Can you work these out from the drawing? Everything is in mm from the part's minimum corner. Round coordinates to 2 decimals unless told otherwise and drop trailing zeros. Write each loop counter-clockwise with the first axis right and the second up, starting at its lowest first coordinate (ties: lowest second). Pieces come first, ordered by that corner, then holes. Notation, with made-up numbers: (-39, 20.5) -> (14, 20.5) arc R28 ccw to (14, 49.5) -> close; hole circle Ø11 at (-11.5, 42.5). An arc over 180 degrees is marked (long way). One line per question, with ' | ' between items. Start each with the question number.
1. Imagine slicing it at B-B, the plane z = 50.8. List the corners of the cut face in (x, y) for me.
2. Imagine slicing it at D-D, the plane x = 64. List the corners of the cut face in (y, z) for me.
3. Imagine slicing it at A-A, the plane x = 38.1. List the corners of the cut face in (y, z) for me, and give its area (3 significant figures).
4. If I drill on line 1 along X through (y, z) = (4.5, 95.25); line 2 along X through (y, z) = (2, 75) (1 decimal); line 3 along X through (y, z) = (2.75, 33.5), over which ranges is the centre line in solid material (lowest first)? Write a range as [from, to].
5. Imagine slicing it at C-C, the plane z = 95.25. List the corners of the cut face in (x, y) for me, and give its area (3 significant figures).
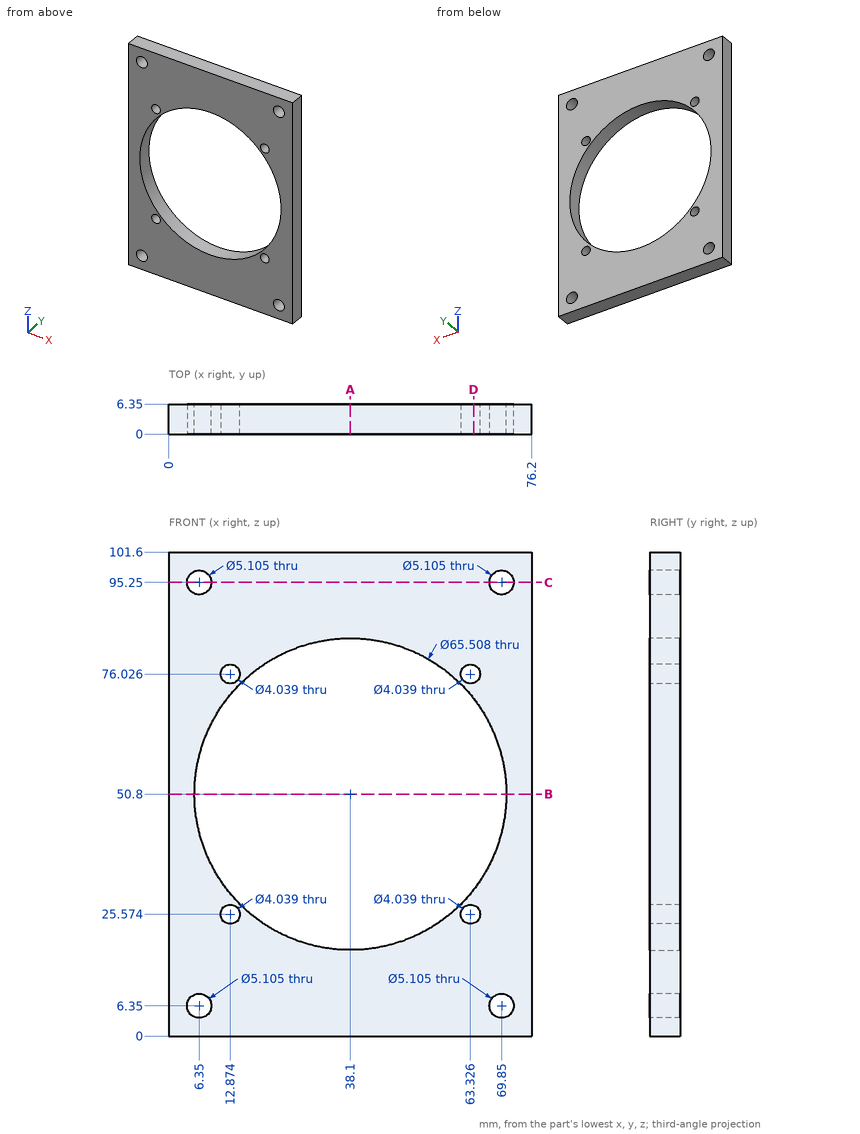
Geometry results:
1) outline: (0, 0) -> (5.35, 0) -> (5.35, 6.35) -> (0, 6.35) -> close; (70.85, 0) -> (76.2, 0) -> (76.2, 6.35) -> (70.85, 6.35) -> close
2) outline: (0, 0) -> (6.35, 0) -> (6.35, 23.67) -> (0, 23.67) -> close; (0, 27.48) -> (6.35, 27.48) -> (6.35, 30.75) -> (0, 30.75) -> close; (0, 70.85) -> (6.35, 70.85) -> (6.35, 74.12) -> (0, 74.12) -> close; (0, 77.93) -> (6.35, 77.93) -> (6.35, 101.6) -> (0, 101.6) -> close
3) outline: (0, 0) -> (6.35, 0) -> (6.35, 18.05) -> (0, 18.05) -> close; (0, 83.55) -> (6.35, 83.55) -> (6.35, 101.6) -> (0, 101.6) -> close | area: 229 mm2
4) line 1: x = [0, 3.8], [8.9, 67.3], [72.4, 76.2] | line 2: x = [0, 11.1], [14.6, 16], [60.2, 61.6], [65.1, 76.2] | line 3: x = [0, 10.29], [65.91, 76.2]
5) outline: (0, 0) -> (3.8, 0) -> (3.8, 6.35) -> (0, 6.35) -> close; (8.9, 0) -> (67.3, 0) -> (67.3, 6.35) -> (8.9, 6.35) -> close; (72.4, 0) -> (76.2, 0) -> (76.2, 6.35) -> (72.4, 6.35) -> close | area: 419 mm2
